Can you work these out from the model? Positions are in its coordinate system, mm. Coordinates: 2 decimals unless noted, no trailing zeros. Order: outer loops, then holes, each group sorted by start corner. A loop starts at its lowest first (then second) coordinate and runs counter-clockwise, first axis right, second up. Notation, with made-up numbers: (81.5, 83.25) -> (137.5, 83.25) arc R20 ccw to (137.5, 119.25) -> close; hole circle Ø6 at (38.5, 43.25). An arc over 180 degrees is marked (long way). Answer as a JSON object with one key per item and string values. Group by question number.
(1) I want a section at A-A, the plane z = 117.5. List the corners of the cut face in (x, y) for me.
(2) For pin 1 (3.5 mm diameter, centred on y = 0, z = 55, fed in from -X), with a flat end and sliding along its axis, tell me the tip position at first contact or that it passes through.
(3) I want a section at B-B, the plane y = 0. List the corners of the cut face in (x, z) for me, plus the area to 3 significant figures.
(4) I need wall thicknesses on line 1 (Z direction, x = 0.25, y = 0); line 2 (Z direction, x = 0.75, y = -0.5). Which ranges of each line are inside material? Lowest first, please.
(5) If we mould it in two halves opening along Z, with no side actions, what happens to faces 1 (the cylindrical face through (0.073, 1.075, 119.186)), 2 (the flat face through (-5.2, 0, 64)), 3 (the flat face through (0, 0, 0))? For each: pulls with the +Z half, pulls with the -Z half, needs draft (parallel to the pull), parting line crosses it, or undercut.
(6) I want a section at C-C, the plane z = 55. List the corners of the cut face in (x, y) for me, plus the area to 3 significant figures.
from build123d import *

# Parameters (mm, degrees)
SKETCH_W        = 10.4
SKETCH_H        = 25
PAD_DEPTH       = 130
SKETCH001_R     = 1.5
POCKET_DEPTH    = 100
SKETCH002_R     = 2
POCKET001_DEPTH = 100


with BuildPart() as part:
    # Sketch → Pad (new body)
    with BuildSketch(Plane.XY):
        Rectangle(SKETCH_W, SKETCH_H)
    extrude(amount=PAD_DEPTH)

    # Sketch001 (on Face2 of Pad) → Pocket (cut)
    with BuildSketch(Plane.YZ.offset(5.2)):
        with Locations((0, 55)):
            Circle(SKETCH001_R)
    extrude(amount=-POCKET_DEPTH, mode=Mode.SUBTRACT)

    # Sketch002 (on Face3 of Pocket) → Pocket001 (cut)
    with BuildSketch(Plane.YZ.offset(5.2)):
        with Locations((0, 117.5)):
            Circle(SKETCH002_R)
    extrude(amount=-POCKET001_DEPTH, mode=Mode.SUBTRACT)


solid = part.part
Computed values:
{
 "1": {"outline": "(-5.2, -12.5) -> (5.2, -12.5) -> (5.2, -2) -> (-5.2, -2) -> close; (-5.2, 2) -> (5.2, 2) -> (5.2, 12.5) -> (-5.2, 12.5) -> close"},
 "2": {"pin 1": "stops at x = -5.2"},
 "3": {"outline": "(-5.2, 0) -> (5.2, 0) -> (5.2, 53.5) -> (-5.2, 53.5) -> close; (-5.2, 56.5) -> (5.2, 56.5) -> (5.2, 115.5) -> (-5.2, 115.5) -> close; (-5.2, 119.5) -> (5.2, 119.5) -> (5.2, 130) -> (-5.2, 130) -> close", "area": "1,280 mm2"},
 "4": {"line 1": "z = 0 to 53.5, 56.5 to 115.5, 119.5 to 130", "line 2": "z = 0 to 53.59, 56.41 to 115.56, 119.44 to 130"},
 "5": {"face 1": "undercut", "face 2": "needs draft", "face 3": "pulls with the -Z half"},
 "6": {"outline": "(-5.2, -12.5) -> (5.2, -12.5) -> (5.2, -1.5) -> (-5.2, -1.5) -> close; (-5.2, 1.5) -> (5.2, 1.5) -> (5.2, 12.5) -> (-5.2, 12.5) -> close", "area": "229 mm2"}
}
